from build123d import *

# Parameters (mm, degrees)
F1_DEPTH    = 9.525
F3_DEPTH    = 25.4
F4_W        = 9.525
F4_H        = 152.4033595958
F5_DEPTH    = 9.525
F6_T1_DEPTH = 9.525


# Not quite as in the source:
# - a fillet or chamfer that OpenCascade refuses, or shapes differently, is made with other operations: its cross-section is extruded or revolved along the edge and cut away or added


with BuildPart() as f1:
    # F0 (on Front) → F1 (new body)
    with BuildSketch(Plane.XZ):
        with BuildLine():
            Line((0, 152.4033595958), (0, 0))
            Line((0, 0), (119.38, 0))
            Line((119.38, 0), (119.38, 152.4033595958))
            ThreePointArc((119.38, 152.4033595958), (122.160179304, 154.9323166344), (123.19, 158.5468))
            Line((123.19, 158.5468), (123.19, 262.382))
            ThreePointArc((123.19, 262.382), (121.1813383054, 267.2313383054), (116.332, 269.24))
            Line((116.332, 269.24), (3.048, 269.24))
            ThreePointArc((3.048, 269.24), (-1.8013383054, 267.2313383054), (-3.81, 262.382))
            Line((-3.81, 262.382), (-3.81, 158.5468))
            ThreePointArc((-3.81, 158.5468), (-2.780179304, 154.9323166344), (0, 152.4033595958))
        make_face()
    extrude(amount=F1_DEPTH)

    # F2 (on face) → F3 (cut)
    with BuildSketch(Plane.XZ.offset(9.525)):
        with BuildLine():
            Line((46.99, 50.8), (46.99, 0))
            Line((46.99, 0), (72.39, 0))
            Line((72.39, 0), (72.39, 50.8))
            ThreePointArc((72.39, 50.8), (59.69, 63.5), (46.99, 50.8))
        make_face()
    extrude(amount=-F3_DEPTH, mode=Mode.SUBTRACT)

    # F4 (on face) → F5 (join)
    with BuildSketch(Plane.XZ.offset(9.525)):
        with Locations((124.1425, 76.2016797979)):
            Rectangle(F4_W, F4_H)
        with Locations((-4.7625, 76.2016797979)):
            Rectangle(F4_W, F4_H)
    extrude(amount=-F5_DEPTH)

    # F6: fillet of radius 6.858 on 2 edges, made by hand

    # F6_s2 → F6_t1 (join)
    with BuildSketch(Plane.XZ):
        with BuildLine():
            ThreePointArc((123.19, 159.1654387879), (124.8101159807, 154.7386188232), (128.905, 152.4033595958))
            Line((128.905, 152.4033595958), (128.7907, 151.7271516766))
            ThreePointArc((128.7907, 151.7271516766), (124.1425, 151.7175595958), (119.38, 151.7175595958))
            Line((119.38, 151.7175595958), (119.0752, 153.0177036362))
            ThreePointArc((119.0752, 153.0177036362), (122.5042, 158.5468), (122.5042, 159.1654387879))
            Line((122.5042, 159.1654387879), (123.19, 159.1654387879))
        make_face()
        with BuildLine():
            ThreePointArc((-9.525, 152.4033595958), (-5.4301159807, 154.7386188232), (-3.81, 159.1654387879))
            Line((-3.81, 159.1654387879), (-3.1242, 159.1654387879))
            ThreePointArc((-3.1242, 159.1654387879), (-3.1242, 158.5468), (0.3048, 153.0177036362))
            Line((0.3048, 153.0177036362), (0, 151.7175595958))
            ThreePointArc((0, 151.7175595958), (-4.7625, 151.7175595958), (-9.4107, 151.7271516766))
            Line((-9.4107, 151.7271516766), (-9.525, 152.4033595958))
        make_face()
    extrude(amount=F6_T1_DEPTH)


solid = f1.part
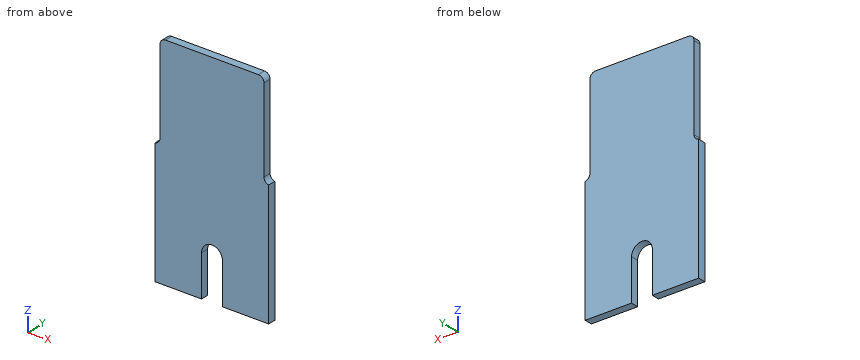
Source: CAD feature listing. Evaluate the final solid. Frame: model axes, mm. Round coordinates to 2 decimals unless told otherwise and drop trailing zeros. Order: outer loops, then holes, each group sorted by start corner. A loop starts at its lowest first (then second) coordinate and runs counter-clockwise, first axis right, second up. Notation, with made-up numbers: (18.5, 47.25) -> (23.5, 47.25) arc R12 ccw to (23.5, 56.25) -> close; hole circle Ø10 at (-20.75, 74). An arc over 180 degrees is marked (long way). Answer as CSV lines item,"result".
Item 1: Section C-C, the plane z = 219. Return loops of the section in (x, y) (3 decimals), plus the area to 3 significant figures.
A:
outline,"(-3.81, -9.525) -> (123.19, -9.525) -> (123.19, 0) -> (-3.81, 0) -> close"
area,"1,210 mm²"
Item 2: Pin query (flat end, axial travel): pin 1 Ø2 at (y, z) = (-8, 188.5) entering from -X. Return the tip coordinate at first contact, or that it passes through.
A:
pin 1,"x = -3.81"
Item 3: Section B-B, the plane y = -4.25. Return loops of the section in (x, z) (3 decimals).
A:
outline,"(-9.525, 0) -> (46.99, 0) -> (46.99, 50.8) arc R12.7 cw to (72.39, 50.8) -> (72.39, 0) -> (128.905, 0) -> (128.905, 152.403) arc R6.858 cw to (123.19, 159.165) -> (123.19, 262.382) arc R6.858 ccw to (116.332, 269.24) -> (3.048, 269.24) arc R6.858 ccw to (-3.81, 262.382) -> (-3.81, 159.165) arc R6.858 cw to (-9.525, 152.403) -> close"
Item 4: Line query: L1, parallel to X at y = -4.5, z = 31 (3 decimals); L2, parallel to X at y = -7.25, z = 246.5; L3, parallel to Z at x = 69, y = -7.5. Output: solid intervals per line, ascending.
A:
L1,"-9.525 to 46.99, 72.39 to 128.905"
L2,"-3.81 to 123.19"
L3,"59.44 to 269.24"
Item 5: Section D-D, the plane x = 59.69. Return loops of the section in (y, z) (3 decimals), plus the area to 3 significant figures.
A:
outline,"(-9.525, 63.5) -> (0, 63.5) -> (0, 269.24) -> (-9.525, 269.24) -> close"
area,"1,960 mm²"
Item 6: Section A-A, the plane z = 58.5. Return loops of the section in (x, y) (1 decimal).
A:
outline,"(-9.5, -9.5) -> (49.6, -9.5) -> (49.6, 0) -> (-9.5, 0) -> close; (69.8, -9.5) -> (128.9, -9.5) -> (128.9, 0) -> (69.8, 0) -> close"
